Check sheet for the modelled part. Datum: model origin and axes. Units: mm. Face numbers are marked on the shaded views. Give positions to 0.01 mm unless a question says otherwise; leave off trailing zeros. Loops run counter-clockwise (first coordinate to the right, second up) from the corner with the lowest first, then second, coordinate; pieces in that order, holes last. Notation, with made-up numbers: (39.5, -36.75) - (72.5, -36.75) arc R31 cw to (72.5, -0.75) - close; hole circle Ø11 at (56.25, 2.5). An arc over 180 degrees is marked (long way). Use CSV: the item, a comma, the result in double quotes.
from build123d import *

# Parameters (mm, degrees)
SKETCH1_R                 = 2.045
BOSS_EXTRUDE1_DEPTH       = 1.524
SKETCH2_R                 = 2.7813
BOSS_EXTRUDE2_DEPTH       = 3.175
F_4_40_TAPPED_HOLE1_D     = 2.2606
F_4_40_TAPPED_HOLE1_DEPTH = 7.62
F_4_40_TAPPED_HOLE1_TIP   = 0.679152758


with BuildPart() as part:
    # Sketch1 → Boss-Extrude1 (new body)
    with BuildSketch(Plane(origin=(0, 0, 0), x_dir=(1, 0, 0), z_dir=(0, 1, 0))):
        Circle(SKETCH1_R)
    extrude(amount=BOSS_EXTRUDE1_DEPTH)

    # Sketch2 → Boss-Extrude2 (add)
    with BuildSketch(Plane(origin=(0, 1.524, 0), x_dir=(1, 0, 0), z_dir=(0, 1, 0))):
        Circle(SKETCH2_R)
    extrude(amount=BOSS_EXTRUDE2_DEPTH)

    # #4-40 Tapped Hole1
    with Locations(Plane(origin=(0, 4.699, 0), x_dir=(1, 0, 0), z_dir=(0, 1, 0))):
        with Locations((0, 0)):
            Hole(F_4_40_TAPPED_HOLE1_D / 2, depth=F_4_40_TAPPED_HOLE1_DEPTH)
            with Locations((0, 0, -(F_4_40_TAPPED_HOLE1_DEPTH + F_4_40_TAPPED_HOLE1_TIP / 2))):  # 118° drill point
                Cone(0, F_4_40_TAPPED_HOLE1_D / 2, F_4_40_TAPPED_HOLE1_TIP, mode=Mode.SUBTRACT)


solid = part.part
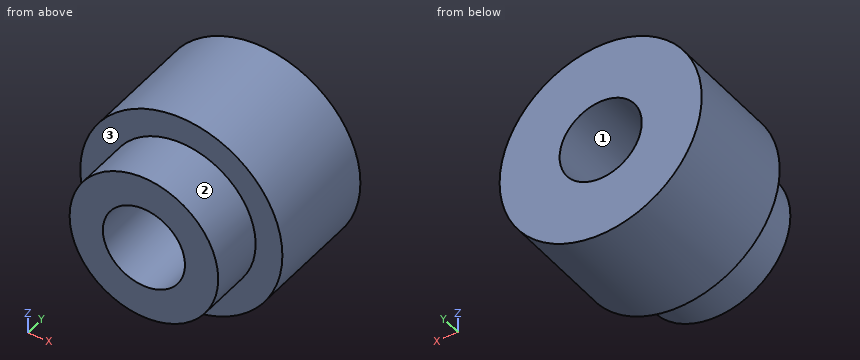
1. Sectioned sample at A-A, the plane x = 0. Record the boundary of the cut face in (y, z) (3 decimals).
Completed:
outline,"(0, -2.045) - (1.524, -2.045) - (1.524, -2.781) - (4.699, -2.781) - (4.699, -1.13) - (0, -1.13) - close; (0, 1.13) - (4.699, 1.13) - (4.699, 2.781) - (1.524, 2.781) - (1.524, 2.045) - (0, 2.045) - close"
2. Go/stop test with flat-tipped pins: pin 1 Ø1.8 at (x, z) = (0, 0) entering from -Y; pin 2 Ø2 at (y, z) = (2.5, 1.5) entering from -X. Record where each tip stops, or that it passes through.
Completed:
pin 1,"passes through"
pin 2,"stops at x = -2.74"
3. Sectioned sample at B-B, the plane z = 0. Record the boundary of the cut face in (x, y) (3 decimals), and give its area (3 significant figures).
Completed:
outline,"(-2.781, 1.524) - (-2.045, 1.524) - (-2.045, 0) - (-1.13, 0) - (-1.13, 4.699) - (-2.781, 4.699) - close; (1.13, 0) - (2.045, 0) - (2.045, 1.524) - (2.781, 1.524) - (2.781, 4.699) - (1.13, 4.699) - close"
area,"13.3 mm²"
4. Sectioned sample at C-C, the plane y = 3.7. Record the boundary of the cut face in (x, z), and give its area (3 significant figures).
Completed:
outline,"circle Ø5.56 at (0, 0); hole circle Ø2.26 at (0, 0)"
area,"20.3 mm²"
5. Release check for a two-part mould opening along Z. For the marked faces 1, 2 and 3 record: released by +Z, released by -Z, zero draft, split by the parting line, or undercut.
Completed:
face 1,"undercut"
face 2,"split by the parting line"
face 3,"zero draft"
6. Scan lines: line 1 along Z through (x, y) = (0, 2.55); line 2 along Y through (x, z) = (0.35, -2.3); line 3 along X through (y, z) = (0.9, -0.35). Record each from-to range of solid material in increasing order.
Completed:
line 1,"z = -2.78 to -1.13, 1.13 to 2.78"
line 2,"y = 1.52 to 4.7"
line 3,"x = -2.01 to -1.07, 1.07 to 2.01"
7. Sectioned sample at D-D, the plane z = -1.5. Record the boundary of the cut face in (x, y).
Completed:
outline,"(-2.34, 1.52) - (-1.39, 1.52) - (-1.39, 0) - (1.39, 0) - (1.39, 1.52) - (2.34, 1.52) - (2.34, 4.7) - (-2.34, 4.7) - close"
